Verification items for the finished model (mm, model axes). Coordinates: 2 decimals unless noted, no trailing zeros. Loops run counter-clockwise (first coordinate to the right, second up) from the corner with the lowest first, then second, coordinate; pieces in that order, holes last. Notation, with made-up numbers: (19.5, 54) -> (60.5, 54) arc R15 ccw to (60.5, 76) -> close; hole circle Ø1 at (-33.5, 27). An arc over 180 degrees is marked (long way). Write item = value, one per line.
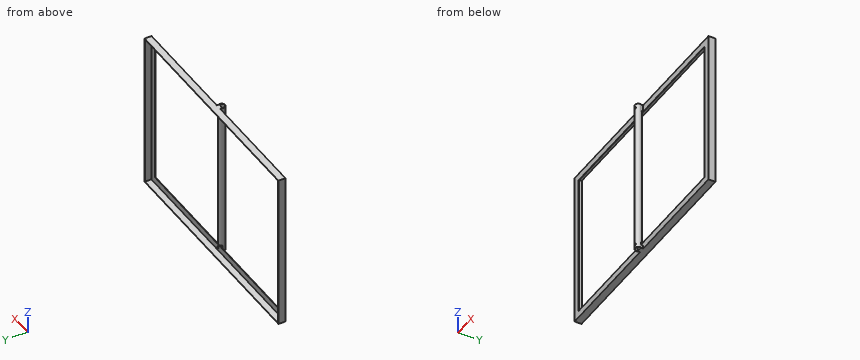
```python
from build123d import *

# Parameters (mm, degrees)
SKETCH2_R            = 14
SKETCH2_R_2          = 12.5
BOSS_EXTRUDE3_DEPTH  = 800
SKETCH3_W            = 50.702600358
SKETCH3_H            = 14.280844995
CUT_EXTRUDE2_DEPTH   = 800
SKETCH5_W            = 25
SKETCH5_H            = 30
BOSS_EXTRUDE4_DEPTH  = 10
SKETCH7_W            = 990
SKETCH7_H            = 685
SKETCH7_W_2          = 930
SKETCH7_H_2          = 625
BOSS_EXTRUDE7_DEPTH  = 30
SKETCH8_W            = 986
SKETCH8_H            = 681
CUT_EXTRUDE3_DEPTH   = 28
SKETCH9_R            = 5
CUT_EXTRUDE4_DEPTH   = 40
SKETCH15_W           = 1140
SKETCH15_H           = 860
SKETCH15_W_2         = 980
SKETCH15_H_2         = 700
CUT_EXTRUDE6_DEPTH   = 149
SKETCH17_W           = 10
SKETCH17_H           = 2
BOSS_EXTRUDE11_DEPTH = 685
SKETCH20_W           = 25
SKETCH20_H           = 15
CUT_EXTRUDE7_DEPTH   = 38
SKETCH22_R           = 14
SKETCH22_R_2         = 12.5
BOSS_EXTRUDE13_DEPTH = 627
SKETCH23_W           = 59.046620232
SKETCH23_H           = 45.176343133
CUT_EXTRUDE8_DEPTH   = 627


with BuildPart() as part:
    # Sketch2 → Boss-Extrude3 (new body)
    with BuildSketch(Plane.XY):
        with Locations((-96.233955608, 31.778750266)):
            Circle(SKETCH2_R)
        with Locations((-96.233955608, 31.778750266)):
            Circle(SKETCH2_R_2, mode=Mode.SUBTRACT)
    extrude(amount=BOSS_EXTRUDE3_DEPTH)

    # Sketch3 → Cut-Extrude2 (cut)
    with BuildSketch(Plane.XY.offset(800)):
        with Locations((-97.127751448, 43.123650815)):
            Rectangle(SKETCH3_W, SKETCH3_H)
    extrude(amount=-CUT_EXTRUDE2_DEPTH, mode=Mode.SUBTRACT)

    # Sketch5 → Boss-Extrude4 (add)
    with BuildSketch(Plane(origin=(0, 35.983228318, 0), x_dir=(1, 0, 0), z_dir=(0, 1, 0))):
        with Locations((-96.233955608, -65)):
            Rectangle(SKETCH5_W, SKETCH5_H)
        with Locations((-96.233955608, -735)):
            Rectangle(SKETCH5_W, SKETCH5_H)
    extrude(amount=BOSS_EXTRUDE4_DEPTH)

    # Sketch7 → Boss-Extrude7 (add)
    with BuildSketch(Plane(origin=(0, 45.983228318, 0), x_dir=(1, 0, 0), z_dir=(0, 1, 0))):
        with Locations((-96.233955608, -407.5)):
            Rectangle(SKETCH7_W, SKETCH7_H)
        with Locations((-96.233955608, -407.5)):
            Rectangle(SKETCH7_W_2, SKETCH7_H_2, mode=Mode.SUBTRACT)
    extrude(amount=BOSS_EXTRUDE7_DEPTH)

    # Sketch8 → Cut-Extrude3 (cut)
    with BuildSketch(Plane(origin=(0, 75.983228318, 0), x_dir=(1, 0, 0), z_dir=(0, 1, 0))):
        with Locations((-96.233955608, -407.5)):
            Rectangle(SKETCH8_W, SKETCH8_H)
    extrude(amount=-CUT_EXTRUDE3_DEPTH, mode=Mode.SUBTRACT)

    # Sketch9 → Cut-Extrude4 (cut)
    with BuildSketch(Plane(origin=(0, 47.983228318, 0), x_dir=(1, 0, 0), z_dir=(0, 1, 0))):
        with Locations((-96.432449353, -82)):
            Circle(SKETCH9_R)
        with Locations((-96.432449353, -733)):
            Circle(SKETCH9_R)
    extrude(amount=-CUT_EXTRUDE4_DEPTH, mode=Mode.SUBTRACT)

    # Sketch15 → Cut-Extrude6 (cut)
    with BuildSketch(Plane(origin=(0, 47.983228318, 0), x_dir=(1, 0, 0), z_dir=(0, 1, 0))):
        with Locations((-91.233955608, -400)):
            Rectangle(SKETCH15_W, SKETCH15_H)
        with Locations((-91.233955608, -400)):
            Rectangle(SKETCH15_W_2, SKETCH15_H_2, mode=Mode.SUBTRACT)
    extrude(amount=-CUT_EXTRUDE6_DEPTH, mode=Mode.SUBTRACT)

    # Sketch17 → Boss-Extrude11 (add)
    with BuildSketch(Plane.XY.offset(750)):
        with Locations((-586.233955608, 46.983228318)):
            Rectangle(SKETCH17_W, SKETCH17_H)
    extrude(amount=-BOSS_EXTRUDE11_DEPTH)

    # Sketch20 → Cut-Extrude7 (cut)
    with BuildSketch(Plane(origin=(0, 45.983228318, 0), x_dir=(1, 0, 0), z_dir=(0, 1, 0))):
        with Locations((-96.233955608, -57.5)):
            Rectangle(SKETCH20_W, SKETCH20_H)
    extrude(amount=-CUT_EXTRUDE7_DEPTH, mode=Mode.SUBTRACT)

    # Sketch22 → Boss-Extrude13 (add)
    with BuildSketch(Plane(origin=(0, 0, 720), x_dir=(-1, 0, 0), z_dir=(0, 0, -1))):
        with Locations((96.233955608, 31.778750266)):
            Circle(SKETCH22_R)
        with Locations((96.233955608, 31.778750266)):
            Circle(SKETCH22_R_2, mode=Mode.SUBTRACT)
    extrude(amount=BOSS_EXTRUDE13_DEPTH)

    # Sketch23 → Cut-Extrude8 (cut)
    with BuildSketch(Plane(origin=(0, 47.983228318, 0), x_dir=(1, 0, 0), z_dir=(0, 1, 0))):
        with Locations((-102.636866369, -42.411828433)):
            Rectangle(SKETCH23_W, SKETCH23_H)
    extrude(amount=-CUT_EXTRUDE8_DEPTH, mode=Mode.SUBTRACT)


solid = part.part
```
1) Depth check by flat-ended pin: pin 1 Ø1 at (y, z) = (24, 154.5) entering from -X; pin 2 Ø0.8 at (x, z) = (-109, 74) entering from +Y; pin 3 Ø3 at (y, z) = (43, 69.5) entering from +X. Enter the tip coordinate at first touch or a pass-through.
Ans:
pin_1 = -108.19
pin_2 = 47.98
pin_3 = -83.73
2) Material ranges on line 1 (Z direction, x = -210, y = 59); line 2 (X direction, y = 55, z = 391.5); line 3 (X direction, y = 36.5, z = 250), recorded low to high.
Ans:
line_1 = 65 to 67, 748 to 750
line_2 = -591.23 to -589.23, 396.77 to 398.77
line_3 = -109.41 to -107.81, -84.66 to -83.05
3) Sectioned sample at B-B, the plane y = 58.5. Record the cut outline in (x, z).
Ans:
outline = (-591.23, 65) -> (398.77, 65) -> (398.77, 750) -> (-591.23, 750) -> close; hole (-589.23, 67) -> (396.77, 67) -> (396.77, 748) -> (-589.23, 748) -> close
4) Sectioned sample at A-A, the plane z = 552.5. Record the cut outline in (x, y), plus the area to 3 significant figures.
Ans:
outline = (-591.23, 45.98) -> (-561.23, 45.98) -> (-561.23, 47.98) -> (-589.23, 47.98) -> (-589.23, 75.98) -> (-591.23, 75.98) -> close; circle Ø28 at (-96.23, 31.78); (368.77, 45.98) -> (398.77, 45.98) -> (398.77, 75.98) -> (396.77, 75.98) -> (396.77, 47.98) -> (368.77, 47.98) -> close; hole circle Ø25 at (-96.23, 31.78)
area = 357 mm2
5) Sectioned sample at C-C, the plane x = -149. Record the cut outline in (y, z).
Ans:
outline = (45.98, 65) -> (75.98, 65) -> (75.98, 67) -> (47.98, 67) -> (47.98, 95) -> (45.98, 95) -> close; (45.98, 720) -> (47.98, 720) -> (47.98, 748) -> (75.98, 748) -> (75.98, 750) -> (45.98, 750) -> close
